Geometry: final body of the model. Coordinates: model frame, mm. Face numbers are marked on the shaded views. Give positions to 0.01 mm unless a question says otherwise; leave off trailing zeros. Loops run counter-clockwise (first coordinate to the right, second up) from the corner with the lowest first, then second, coordinate; pieces in that order, holes last. Notation, with made-up numbers: (-1, -8.5) - (55, -8.5) arc R16 ccw to (55, -2.5) - close; hole circle Ø7 at (-16.75, 36). An arc over 180 degrees is marked (long way). Answer in a Markdown table with one row per item.
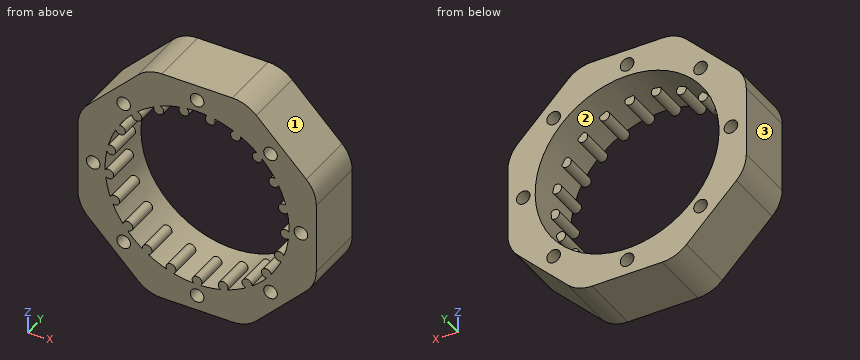
from build123d import *

# Parameters (mm, degrees)
SKETCH1_R           = 32
SKETCH1_R_2         = 27
BOSS_EXTRUDE1_DEPTH = 18
SKETCH2_R           = 1.45
BOSS_EXTRUDE2_DEPTH = 10
SKETCH4_R           = 32
BOSS_EXTRUDE3_DEPTH = 18
SKETCH5_R           = 2
CUT_EXTRUDE2_DEPTH  = 53.668776329
SKETCH3_R           = 2
CUT_EXTRUDE3_DEPTH  = 53.668776329


with BuildPart() as part:
    # Sketch1 → Boss-Extrude1 (new body)
    with BuildSketch(Plane(origin=(0, 0, 0), x_dir=(1, 0, 0), z_dir=(0, 1, 0))):
        with Locations(Location((0, 0, 0), (0, 0, 270))):
            Circle(SKETCH1_R)
        with Locations(Location((0, 0, 0), (0, 0, 270))):
            Circle(SKETCH1_R_2, mode=Mode.SUBTRACT)
    extrude(amount=BOSS_EXTRUDE1_DEPTH)

    # Sketch2 → Boss-Extrude2 (add)
    with BuildSketch(Plane(origin=(0, 0, 0), x_dir=(1, 0, 0), z_dir=(0, 1, 0))):
        with Locations((0, 26)):
            Circle(SKETCH2_R)
        with Locations((7.663634535, 24.84489295)):
            Circle(SKETCH2_R)
        with Locations((14.64632151, 21.482208132)):
            Circle(SKETCH2_R)
        with Locations((20.327618544, 16.210734848)):
            Circle(SKETCH2_R)
        with Locations((24.202717465, 9.498866634)):
            Circle(SKETCH2_R)
        with Locations((25.927298727, 1.942982433)):
            Circle(SKETCH2_R)
        with Locations((25.348125717, -5.785544283)):
            Circle(SKETCH2_R)
        with Locations((22.516660498, -13)):
            Circle(SKETCH2_R)
        with Locations((17.684491182, -19.059348668)):
            Circle(SKETCH2_R)
        with Locations((11.280977217, -23.425190565)):
            Circle(SKETCH2_R)
        with Locations((3.875098921, -25.709601482)):
            Circle(SKETCH2_R)
        with Locations((-3.875098921, -25.709601482)):
            Circle(SKETCH2_R)
        with Locations((-11.280977217, -23.425190565)):
            Circle(SKETCH2_R)
        with Locations((-17.684491182, -19.059348668)):
            Circle(SKETCH2_R)
        with Locations((-22.516660498, -13)):
            Circle(SKETCH2_R)
        with Locations((-25.348125717, -5.785544283)):
            Circle(SKETCH2_R)
        with Locations((-25.927298727, 1.942982433)):
            Circle(SKETCH2_R)
        with Locations((-24.202717465, 9.498866634)):
            Circle(SKETCH2_R)
        with Locations((-20.327618544, 16.210734848)):
            Circle(SKETCH2_R)
        with Locations((-14.64632151, 21.482208132)):
            Circle(SKETCH2_R)
        with Locations((-7.663634535, 24.84489295)):
            Circle(SKETCH2_R)
    extrude(amount=BOSS_EXTRUDE2_DEPTH)

    # Sketch4 → Boss-Extrude3 (add)
    with BuildSketch(Plane(origin=(0, 0, 0), x_dir=(1, 0, 0), z_dir=(0, 1, 0))):
        with BuildLine():
            Line((10.355339059, 35), (-10.355339059, 35))
            ThreePointArc((-10.355339059, 35), (-14.182173383, 34.238795325), (-17.426406871, 32.071067812))
            Line((-17.426406871, 32.071067812), (-32.071067812, 17.426406871))
            ThreePointArc((-32.071067812, 17.426406871), (-34.238795325, 14.182173383), (-35, 10.355339059))
            Line((-35, 10.355339059), (-35, -10.355339059))
            ThreePointArc((-35, -10.355339059), (-34.238795325, -14.182173383), (-32.071067812, -17.426406871))
            Line((-32.071067812, -17.426406871), (-17.426406871, -32.071067812))
            ThreePointArc((-17.426406871, -32.071067812), (-14.182173383, -34.238795325), (-10.355339059, -35))
            Line((-10.355339059, -35), (10.355339059, -35))
            ThreePointArc((10.355339059, -35), (14.182173383, -34.238795325), (17.426406871, -32.071067812))
            Line((17.426406871, -32.071067812), (32.071067812, -17.426406871))
            ThreePointArc((32.071067812, -17.426406871), (34.238795325, -14.182173383), (35, -10.355339059))
            Line((35, -10.355339059), (35, 10.355339059))
            ThreePointArc((35, 10.355339059), (34.238795325, 14.182173383), (32.071067812, 17.426406871))
            Line((32.071067812, 17.426406871), (17.426406871, 32.071067812))
            ThreePointArc((17.426406871, 32.071067812), (14.182173383, 34.238795325), (10.355339059, 35))
        make_face()
        Circle(SKETCH4_R, mode=Mode.SUBTRACT)
    extrude(amount=BOSS_EXTRUDE3_DEPTH)

    # Sketch5 → Cut-Extrude2 (cut, through all)
    with BuildSketch(Plane(origin=(0, 18, 0), x_dir=(1, 0, 0), z_dir=(0, 1, 0))):
        with Locations(Location((-21.566756826, 21.566756826, 0), (0, 0, 270))):
            Circle(SKETCH5_R)
        with Locations(Location((21.566756826, 21.566756826, 0), (0, 0, 270))):
            Circle(SKETCH5_R)
        with Locations(Location((21.566756826, -21.566756826, 0), (0, 0, 270))):
            Circle(SKETCH5_R)
        with Locations(Location((-21.566756826, -21.566756826, 0), (0, 0, 270))):
            Circle(SKETCH5_R)
    extrude(amount=-CUT_EXTRUDE2_DEPTH, mode=Mode.SUBTRACT)

    # Sketch3 → Cut-Extrude3 (cut, through all)
    with BuildSketch(Plane(origin=(0, 18, 0), x_dir=(1, 0, 0), z_dir=(0, 1, 0))):
        with Locations(Location((0, 30.5, 0), (0, 0, 270))):
            Circle(SKETCH3_R)
        with Locations(Location((30.5, 0, 0), (0, 0, 270))):
            Circle(SKETCH3_R)
        with Locations(Location((0, -30.5, 0), (0, 0, 270))):
            Circle(SKETCH3_R)
        with Locations(Location((-30.5, 0, 0), (0, 0, 270))):
            Circle(SKETCH3_R)
    extrude(amount=-CUT_EXTRUDE3_DEPTH, mode=Mode.SUBTRACT)


solid = part.part
Q1. Cut plane D-D (y = 15.75). Give the number of separate pieces and of enclosed holes in the cut face, and give its area (3 significant figures).
Check values:
| item | result |
|---|---|
| separate pieces | 1 |
| enclosed holes | 9 |
| area | 1,650 mm² |
Q2. First-contact query: pin 1 (1.4 mm diameter, centred on x = -11, z = 23.5, fed in from +Y); pin 2 (3.5 mm diameter, centred on x = 21.57, z = 21.57, fed in from +Y); pin 3 (1.5 mm diameter, centred on x = 14, y = 11, fed in from -Z); pin 4 (4 mm diameter, centred on y = 10.5, z = -12.5, fed in from +X). Flat tips, straight axial feed; report the tip coordinate or a pass-through.
Check values:
| item | result |
|---|---|
| pin 1 | y = 10 |
| pin 2 | through |
| pin 3 | z = -34.57 |
| pin 4 | x = 35 |
Q3. Material intervals for line 1 along X through (y, z) = (10.25, 0); line 2 along Z through (x, y) = (-1.5, 11.5); line 3 along Z through (x, y) = (17, 6.5), sorted ascending.
Check values:
| item | result |
|---|---|
| line 1 | -35 to -32.5, -28.5 to -27, 27 to 28.5, 32.5 to 35 |
| line 2 | -35 to -31.82, -29.18 to -26.96, 26.96 to 29.18, 31.82 to 35 |
| line 3 | -32.47 to -20.98, 17.78 to 20.34, 20.98 to 32.47 |
Q4. Cut plane A-A (x = 0). Output: boundary loops of the cut face in (y, z), and give its area (4 significant figures).
Check values:
| item | result |
|---|---|
| outline | (0, -35) - (18, -35) - (18, -32.5) - (0, -32.5) - close; (0, -28.5) - (18, -28.5) - (18, -27) - (10, -27) - (10, -24.55) - (0, -24.55) - close; (0, 27) - (18, 27) - (18, 28.5) - (0, 28.5) - close; (0, 32.5) - (18, 32.5) - (18, 35) - (0, 35) - close |
| area | 168.5 mm² |
Q5. Cut plane B-B (z = -30.5). Output: boundary loops of the cut face in (x, y), and give its area (3 significant figures).
Check values:
| item | result |
|---|---|
| outline | (-19, 0) - (-2, 0) - (-2, 18) - (-19, 18) - close; (2, 0) - (19, 0) - (19, 18) - (2, 18) - close |
| area | 612 mm² |
Q6. Cut plane C-C (x = 30.5). Output: boundary loops of the cut face in (y, z).
Check values:
| item | result |
|---|---|
| outline | (0, -19) - (18, -19) - (18, -2) - (0, -2) - close; (0, 2) - (18, 2) - (18, 19) - (0, 19) - close |
Q7. Draft query along Z for the marked faces 1, 2 and 3. Return one class per face: pulls with the +Z half, pulls with the -Z half, needs draft (parallel to the pull), parting line crosses it, or undercut.
Check values:
| item | result |
|---|---|
| face 1 | pulls with the +Z half |
| face 2 | undercut |
| face 3 | needs draft |
